Solid Edge part; units mm, degrees
sketch "Sketch1" plane through (0, 0, 0) normal (0, 0, 1) x (1, 0, 0)
  line L0 (250, 91) -> (-250, 91)
  line L1 (-250, 91) -> (-250, -91)
  line L2 (-250, -91) -> (250, -91)
  line L3 (250, -91) -> (250, 91)
extrude "Protrusion1" add sketch "Sketch1" along normal blind 15
sketch "Sketch2" plane through (0, 0, 15) normal (0, 0, 1) x (1, 0, 0)
  circle A0 centre (0, -83.5) radius 3.1
  circle A1 centre (150, -83.5) radius 3.1
  circle A2 centre (-150, -83.5) radius 3.1
extrude "ExtrudedCutout_1" cut sketch "Sketch2" against normal blind 150.8777
sketch "Sketch3" plane through (0, 0, 15) normal (0, 0, 1) x (1, 0, 0)
  circle A0 centre (0, -83.5) radius 5.15
  circle A1 centre (150, -83.5) radius 5.15
  circle A2 centre (-150, -83.5) radius 5.15
extrude "ExtrudedCutout_2" cut sketch "Sketch3" against normal blind 6
mirror "Mirror1" about plane through (0, 0, 0) normal (0, -1, 0) of "ExtrudedCutout_2", "ExtrudedCutout_1"
sketch "Sketch4" plane through (0, 0, 15) normal (0, 0, 1) x (1, 0, 0)
  circle A0 centre (242.5, 0) radius 3.1
  circle A1 centre (-242.5, 0) radius 3.1
extrude "Cutout1" cut sketch "Sketch4" against normal up to next
sketch "Sketch5" plane through (0, 0, 15) normal (0, 0, 1) x (1, 0, 0)
  circle A0 centre (242.5, 0) radius 5.15
  circle A1 centre (-242.5, 0) radius 5.15
  dimension "D1" = 242.5
extrude "ExtrudedCutout_4" cut sketch "Sketch5" against normal blind 6
hole "Hole_2" at (220, 61, 15) direction (0, 0, -1) diameter 8.566 end up to next thread major 10.2 thread length 2
Could you check a few things on this model? Use its own coordinates, in mm. A direction names the side the tool comes from. Round coordinates to 2 decimals unless told otherwise and drop trailing zeros. Write each loop counter-clockwise with the first axis right and the second up, starting at its lowest first coordinate (ties: lowest second). Pieces come first, ordered by that corner, then holes.
(1) For pin 1 (5 mm diameter, centred on x = 152, y = 83.5, fed in from +Z), with a flat end and sliding along its axis, tell me the tip position at first contact or that it passes through.
Findings below:
pin 1: stops at z = 9
(2) If I drill on probe 1 along Y at (x, z) = (150, 13.45); probe 2 along X at (y, z) = (83.5, 12); probe 3 along Y at (x, z) = (-151.5, 13.5), over which ranges is the centre line in solid material (lowest first)?
Findings below:
probe 1: y = -91 to -88.65, -78.35 to 78.35, 88.65 to 91
probe 2: x = -250 to -155.15, -144.85 to -5.15, 5.15 to 144.85, 155.15 to 250
probe 3: y = -91 to -88.43, -78.57 to 78.57, 88.43 to 91
(3) Suppose I cut it at A-A on x = 220. Write out the boundary of the cut face in (y, z).
Findings below:
outline: (-91, 0) - (56.72, 0) - (56.72, 15) - (-91, 15) - close; (65.28, 0) - (91, 0) - (91, 15) - (65.28, 15) - close
(4) Which directions (+Z, -Z, +X, -X, +Y, -Y) give clear straight access to the entire face, cutting with the end or side of a thin tool? Please do faces 4 (the face through (-3, 1, 15)), 5 (the face through (-151.116, -88.528, 12.042)).
Findings below:
face 4: +Z, +X, -X, +Y, -Y
face 5: +Z
(5) Thinking about a two-plate mould opening in X: for faces 1 (the face through (-250, 1, 7)), 2 (the face through (3, 91, 7)), 3 (the face through (150, 87, 9)), which applies, +X half, -X half, draft (parallel to the pull), parting line (faces both ways), or undercut?
Findings below:
face 1: -X half
face 2: draft
face 3: undercut
